Read the model definition and answer for the solid it produces. Units are mm, in the model's axes. Face numbers are marked on the shaded views. Give positions to 0.01 mm unless a question says otherwise; leave off trailing zeros. Loops run counter-clockwise (first coordinate to the right, second up) from the corner with the lowest first, then second, coordinate; pieces in that order, holes last. Notation, with made-up numbers: (53, -38.5) - (60, -38.5) arc R23 cw to (60, -15.5) - close; hole circle Ø6 at (8.5, 28). An arc over 180 degrees is marked (long way). Write item = value, one per line.
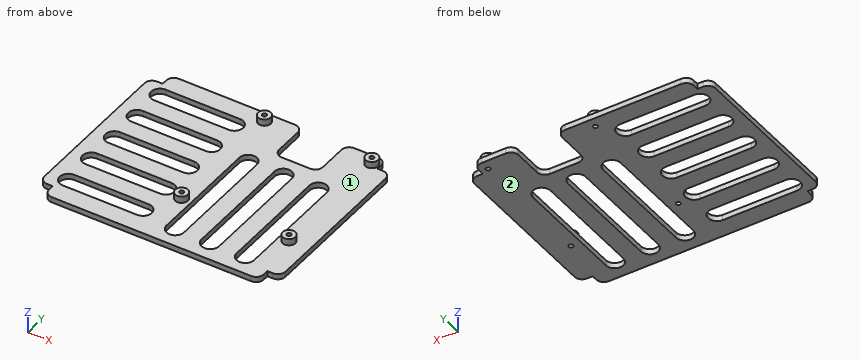
```python
from build123d import *

# Parameters (mm, degrees)
SKETCH_W                           = 110
SKETCH_H                           = 89
PAD_DEPTH                          = 2.5
SKETCH001_R                        = 2.9
PAD001_DEPTH                       = 3
SKETCH002_R                        = 1
POCKET_DEPTH                       = 5.501
SKETCH003_W                        = 20
SKETCH003_H                        = 20
POCKET001_DEPTH                    = 2.501
POCKET002_DEPTH                    = 285.705873
POCKET002_LINEARPATTERN_2_DEPTH    = 285.705873
LINEARPATTERN001_COUNT             = 2
LINEARPATTERN001_PITCH             = 16
POCKET003_DEPTH                    = 285.705873
POCKET003_LINEARPATTERN002_2_DEPTH = 285.705873
POCKET003_LINEARPATTERN002_3_DEPTH = 285.705873
LINEARPATTERN003_COUNT             = 3
LINEARPATTERN003_PITCH             = 16
FILLET_R                           = 3.5
SKETCH006_W                        = 6
SKETCH006_H                        = 6
POCKET004_DEPTH                    = 285.705873
FILLET001_R                        = 3.5


with BuildPart() as part:
    # Sketch → Pad (new body)
    with BuildSketch(Plane.XY):
        with Locations((55, 0)):
            Rectangle(SKETCH_W, SKETCH_H)
    extrude(amount=PAD_DEPTH)

    # Sketch001 (on Face6 of Pad) → Pad001 (join)
    with BuildSketch(Plane.XY.offset(2.5)):
        with Locations((100.5, 40)):
            Circle(SKETCH001_R)
        with Locations((100.5, -18)):
            Circle(SKETCH001_R)
        with Locations((51.5, 40)):
            Circle(SKETCH001_R)
        with Locations((51.5, -18)):
            Circle(SKETCH001_R)
    extrude(amount=PAD001_DEPTH)

    # Sketch002 (on Face13 of Pad001) → Pocket (cut, through all)
    with BuildSketch(Plane.XY.offset(5.5)):
        with Locations((51.5, 40)):
            Circle(SKETCH002_R)
        with Locations((100.5, 40)):
            Circle(SKETCH002_R)
        with Locations((51.5, -18)):
            Circle(SKETCH002_R)
        with Locations((100.5, -18)):
            Circle(SKETCH002_R)
    extrude(amount=-POCKET_DEPTH, mode=Mode.SUBTRACT)

    # Sketch003 → Pocket001 (cut, through all)
    with BuildSketch(Plane.XY.offset(2.5)):
        with Locations((76, 34.5)):
            Rectangle(SKETCH003_W, SKETCH003_H)
    extrude(amount=-POCKET001_DEPTH, mode=Mode.SUBTRACT)

    # Sketch004 (on Face5 of Pocket001) → Pocket002 (cut, through all)
    with BuildSketch(Plane.XY.offset(2.5)):
        with BuildLine():
            ThreePointArc((80, 15.5), (76, 19.5), (72, 15.5))
            Line((72, 15.5), (72, -35.5))
            ThreePointArc((72, -35.5), (76, -39.5), (80, -35.5))
            Line((80, 15.5), (80, -35.5))
        make_face()
    pocket002 = extrude(amount=-POCKET002_DEPTH, mode=Mode.SUBTRACT)

    # Sketch004 LinearPattern 2 → Pocket002 LinearPattern 2 (cut, through all)
    with BuildSketch(Plane(origin=(16, 0, 2.5), x_dir=(1, 0, 0), z_dir=(0, 0, 1))):
        with BuildLine():
            ThreePointArc((80, 15.5), (76, 19.5), (72, 15.5))
            Line((72, 15.5), (72, -35.5))
            ThreePointArc((72, -35.5), (76, -39.5), (80, -35.5))
            Line((80, 15.5), (80, -35.5))
        make_face()
    pocket002_linearpattern_2 = extrude(amount=-POCKET002_LINEARPATTERN_2_DEPTH, mode=Mode.SUBTRACT)

    # LinearPattern001: Pocket002, Pocket002 LinearPattern 2 ×2
    with Locations(*[(-i * LINEARPATTERN001_PITCH, 0, 0) for i in range(1, LINEARPATTERN001_COUNT)]):
        add(pocket002, mode=Mode.SUBTRACT)
        add(pocket002_linearpattern_2, mode=Mode.SUBTRACT)

    # Sketch005 (on Face5 of MultiTransform) → Pocket003 (cut, through all)
    with BuildSketch(Plane.XY.offset(2.5)):
        with BuildLine():
            ThreePointArc((9, 4), (5, 0), (9, -4))
            Line((9, -4), (43, -4))
            ThreePointArc((43, -4), (47, 0), (43, 4))
            Line((9, 4), (43, 4))
        make_face()
    pocket003 = extrude(amount=-POCKET003_DEPTH, mode=Mode.SUBTRACT)

    # Sketch005 LinearPattern002 2 → Pocket003 LinearPattern002 2 (cut, through all)
    with BuildSketch(Plane(origin=(0, 16, 2.5), x_dir=(1, 0, 0), z_dir=(0, 0, 1))):
        with BuildLine():
            ThreePointArc((9, 4), (5, 0), (9, -4))
            Line((9, -4), (43, -4))
            ThreePointArc((43, -4), (47, 0), (43, 4))
            Line((9, 4), (43, 4))
        make_face()
    pocket003_linearpattern002_2 = extrude(amount=-POCKET003_LINEARPATTERN002_2_DEPTH, mode=Mode.SUBTRACT)

    # Sketch005 LinearPattern002 3 → Pocket003 LinearPattern002 3 (cut, through all)
    with BuildSketch(Plane(origin=(0, 32, 2.5), x_dir=(1, 0, 0), z_dir=(0, 0, 1))):
        with BuildLine():
            ThreePointArc((9, 4), (5, 0), (9, -4))
            Line((9, -4), (43, -4))
            ThreePointArc((43, -4), (47, 0), (43, 4))
            Line((9, 4), (43, 4))
        make_face()
    pocket003_linearpattern002_3 = extrude(amount=-POCKET003_LINEARPATTERN002_3_DEPTH, mode=Mode.SUBTRACT)

    # LinearPattern003: Pocket003, Pocket003 LinearPattern002 2, Pocket003 LinearPattern002 3 ×3
    with Locations(*[(0, -i * LINEARPATTERN003_PITCH, 0) for i in range(1, LINEARPATTERN003_COUNT)]):
        add(pocket003, mode=Mode.SUBTRACT)
        add(pocket003_linearpattern002_2, mode=Mode.SUBTRACT)
        add(pocket003_linearpattern002_3, mode=Mode.SUBTRACT)

    # Fillet
    fillet_edges = [part.edges().sort_by_distance(p)[0] for p in [
        (110, 44.5, 1.25),
        (66, 44.5, 1.25),
        (66, 24.5, 1.25),
        (110, -44.5, 1.25),
        (86, 44.5, 1.25),
        (86, 24.5, 1.25),
        (0, 44.5, 1.25),
        (0, -44.5, 1.25),
    ]]
    fillet(fillet_edges, radius=FILLET_R)

    # Sketch006 (on Face5 of Fillet) → Pocket004 (cut, through all)
    with BuildSketch(Plane.XY.offset(2.5)):
        with Locations((3, 41.5)):
            Rectangle(SKETCH006_W, SKETCH006_H)
        with Locations((107, 41.5)):
            Rectangle(SKETCH006_W, SKETCH006_H)
    pocket004 = extrude(amount=-POCKET004_DEPTH, mode=Mode.SUBTRACT)

    # Mirrored: Pocket004 across XZ
    add(pocket004.mirror(Plane.XZ), mode=Mode.SUBTRACT)

    # Fillet001
    fillet001_edges = [part.edges().sort_by_distance(p)[0] for p in [
        (6, 44.5, 1.25),
        (0, 38.5, 1.25),
        (104, 44.5, 1.25),
        (110, 38.5, 1.25),
        (110, -38.5, 1.25),
        (104, -44.5, 1.25),
        (6, -44.5, 1.25),
        (0, -38.5, 1.25),
    ]]
    fillet(fillet001_edges, radius=FILLET001_R)


solid = part.part
```
1) The mould has two halves that part along Y. Classify the marked faces 1 and 2: pulls with the +Y half, pulls with the -Y half, needs draft (parallel to the pull), parting line crosses it, or undercut.
Output:
face_1 = undercut
face_2 = needs draft
2) A cutting plane is placed at B-B on x = 36.5. Determine the outline of the cut face in (y, z), then the cut area to 4 significant figures.
Output:
outline = (-44.5, 0) - (-36, 0) - (-36, 2.5) - (-44.5, 2.5) - close; (-28, 0) - (-20, 0) - (-20, 2.5) - (-28, 2.5) - close; (-12, 0) - (-4, 0) - (-4, 2.5) - (-12, 2.5) - close; (4, 0) - (12, 0) - (12, 2.5) - (4, 2.5) - close; (20, 0) - (28, 0) - (28, 2.5) - (20, 2.5) - close; (36, 0) - (44.5, 0) - (44.5, 2.5) - (36, 2.5) - close
area = 122.5 mm²
3) Find the intervals of material crossed by probe 1 along Y at (x, z) = (100.5, 2.2); probe 2 along Y at (x, z) = (100.5, 4.15); probe 3 along Y at (x, z) = (10, 1.75), in increasing order.
Output:
probe_1 = -44.5 to -19, -17 to 39, 41 to 44.5
probe_2 = -20.9 to -19, -17 to -15.1, 37.1 to 39, 41 to 42.9
probe_3 = -44.5 to -36, -28 to -20, -12 to -4, 4 to 12, 20 to 28, 36 to 44.5
4) A cutting plane is placed at C-C on y = -32. Determine the outline of the cut face in (x, z), then the cut area to 3 significant figures.
Output:
outline = (0, 0) - (5, 0) - (5, 2.5) - (0, 2.5) - close; (47, 0) - (56, 0) - (56, 2.5) - (47, 2.5) - close; (64, 0) - (72, 0) - (72, 2.5) - (64, 2.5) - close; (80, 0) - (88, 0) - (88, 2.5) - (80, 2.5) - close; (96, 0) - (110, 0) - (110, 2.5) - (96, 2.5) - close
area = 110 mm²
5) A cutting plane is placed at D-D on x = 91. Determine the outline of the cut face in (y, z).
Output:
outline = (-44.5, 0) - (-39.37, 0) - (-39.37, 2.5) - (-44.5, 2.5) - close; (19.37, 0) - (44.5, 0) - (44.5, 2.5) - (19.37, 2.5) - close
6) A cutting plane is placed at A-A on z = 4.45. Determine the outline of the cut face in (x, y), then the cut area to 3 significant figures.
Output:
outline = circle Ø5.8 at (51.5, -18); circle Ø5.8 at (51.5, 40); circle Ø5.8 at (100.5, -18); circle Ø5.8 at (100.5, 40); hole circle Ø2 at (51.5, -18); hole circle Ø2 at (51.5, 40); hole circle Ø2 at (100.5, -18); hole circle Ø2 at (100.5, 40)
area = 93.1 mm²
7) Each of these flat-tipped pins is pushed along its axis until it touches: P1, Ø3, axis at x = 24, z = 4.5, coming from the +Y side; P2, Ø1.2, axis at y = 40, z = 1.5, coming from the +X side; P3, Ø1, axis at x = 51.5, z = 4, coming from the +Y side; P4, Ø2, axis at x = 106, z = 0.5, coming from the -Y side. Where does it stop, or does it pass through?
Output:
P1 = through
P2 = 104
P3 = 42.9
P4 = -38.5
